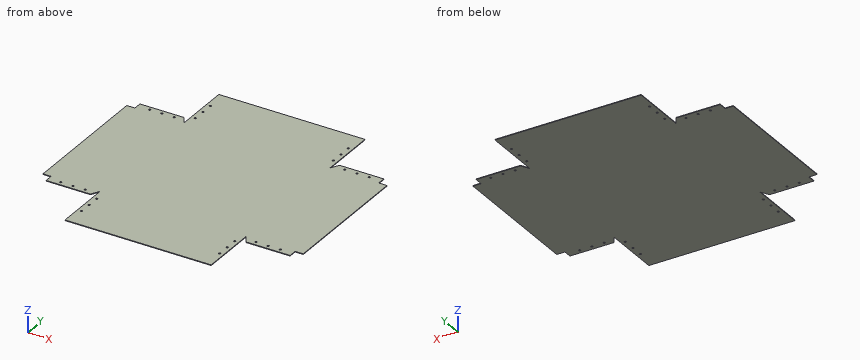
```python
from build123d import *

# Parameters (mm, degrees)
F0_W     = 227.80625
F0_H     = 12.7
F0_W_2   = 6.35
F0_H_2   = 212.725
F0_W_3   = 76.2
F0_R     = 1.5875
F1_DEPTH = 0.508


with BuildPart() as f1:
    # F0 (on Top) → F1 (new body, symmetric)
    with BuildSketch(Plane.XY):
        with Locations((0, -188.9125)):
            Rectangle(F0_W, F0_H)
        with Locations((-199.628125, 0)):
            Rectangle(F0_W_2, F0_H_2)
        with Locations((199.628125, 0)):
            Rectangle(F0_W_2, F0_H_2)
        Polygon((-107.553125, 182.5625), (113.903125, 182.5625), (113.903125, 195.2625), (-113.903125, 195.2625), (-113.903125, 182.5625), align=None)
        with Locations((-193.278125, 0)):
            Rectangle(F0_W_2, F0_H_2)
        with Locations((193.278125, 0)):
            Rectangle(F0_W_2, F0_H_2)
        with Locations((152.003125, 0)):
            Rectangle(F0_W_3, F0_H_2)
        with Locations((-152.003125, 0)):
            Rectangle(F0_W_3, F0_H_2)
        Polygon((-121.235473, -119.0625), (-113.903125, -106.3625), (-190.103125, -106.3625), (-190.103125, -119.0625), align=None)
        with Locations((-171.053125, -112.7125)):
            Circle(F0_R, mode=Mode.SUBTRACT)
        with Locations((-152.003125, -112.7125)):
            Circle(F0_R, mode=Mode.SUBTRACT)
        with Locations((-132.953125, -112.7125)):
            Circle(F0_R, mode=Mode.SUBTRACT)
        with BuildLine():
            Line((-131.365625, 112.7125), (-117.569299, 112.7125))
            Line((-117.569299, 112.7125), (-121.235473, 119.0625))
            Line((-121.235473, 119.0625), (-190.103125, 119.0625))
            Line((-190.103125, 119.0625), (-190.103125, 112.7125))
            Line((-190.103125, 112.7125), (-172.640625, 112.7125))
            ThreePointArc((-172.640625, 112.7125), (-171.053125, 114.3), (-169.465625, 112.7125))
            Line((-169.465625, 112.7125), (-153.590625, 112.7125))
            ThreePointArc((-153.590625, 112.7125), (-152.003125, 114.3), (-150.415625, 112.7125))
            Line((-150.415625, 112.7125), (-134.540625, 112.7125))
            ThreePointArc((-134.540625, 112.7125), (-132.953125, 114.3), (-131.365625, 112.7125))
        make_face()
        Polygon((190.103125, -106.3625), (113.903125, -106.3625), (121.235473, -119.0625), (190.103125, -119.0625), align=None)
        with Locations((132.953125, -112.7125)):
            Circle(F0_R, mode=Mode.SUBTRACT)
        with Locations((152.003125, -112.7125)):
            Circle(F0_R, mode=Mode.SUBTRACT)
        with Locations((171.053125, -112.7125)):
            Circle(F0_R, mode=Mode.SUBTRACT)
        Polygon((121.235473, 119.0625), (113.903125, 106.3625), (190.103125, 106.3625), (190.103125, 119.0625), align=None)
        with Locations((132.953125, 112.7125)):
            Circle(F0_R, mode=Mode.SUBTRACT)
        with Locations((152.003125, 112.7125)):
            Circle(F0_R, mode=Mode.SUBTRACT)
        with Locations((171.053125, 112.7125)):
            Circle(F0_R, mode=Mode.SUBTRACT)
        with BuildLine():
            Line((-190.103125, 106.3625), (-113.903125, 106.3625))
            Line((-113.903125, 106.3625), (-117.569299, 112.7125))
            Line((-117.569299, 112.7125), (-131.365625, 112.7125))
            ThreePointArc((-131.365625, 112.7125), (-132.953125, 111.125), (-134.540625, 112.7125))
            Line((-134.540625, 112.7125), (-150.415625, 112.7125))
            ThreePointArc((-150.415625, 112.7125), (-152.003125, 111.125), (-153.590625, 112.7125))
            Line((-153.590625, 112.7125), (-169.465625, 112.7125))
            ThreePointArc((-169.465625, 112.7125), (-171.053125, 111.125), (-172.640625, 112.7125))
            Line((-172.640625, 112.7125), (-190.103125, 112.7125))
            Line((-190.103125, 112.7125), (-190.103125, 106.3625))
        make_face()
        with BuildLine():
            Line((-113.903125, 106.3625), (-107.553125, 106.3625))
            Line((-107.553125, 106.3625), (-107.553125, 123.825))
            ThreePointArc((-107.553125, 123.825), (-109.140625, 125.4125), (-107.553125, 127))
            Line((-107.553125, 127), (-107.553125, 142.875))
            ThreePointArc((-107.553125, 142.875), (-109.140625, 144.4625), (-107.553125, 146.05))
            Line((-107.553125, 146.05), (-107.553125, 161.925))
            ThreePointArc((-107.553125, 161.925), (-109.140625, 163.5125), (-107.553125, 165.1))
            Line((-107.553125, 165.1), (-107.553125, 182.5625))
            Line((-107.553125, 182.5625), (-113.903125, 182.5625))
            Line((-113.903125, 182.5625), (-113.903125, 119.0625))
            Line((-113.903125, 119.0625), (-113.903125, 112.7125))
            Line((-113.903125, 112.7125), (-113.903125, 106.3625))
        make_face()
        Polygon((113.903125, -119.0625), (113.903125, -106.3625), (-113.903125, -106.3625), (-113.903125, -119.0625), (-113.903125, -182.5625), (113.903125, -182.5625), align=None)
        with Locations((-107.553125, -163.5125)):
            Circle(F0_R, mode=Mode.SUBTRACT)
        with Locations((-107.553125, -144.4625)):
            Circle(F0_R, mode=Mode.SUBTRACT)
        with Locations((-107.553125, -125.4125)):
            Circle(F0_R, mode=Mode.SUBTRACT)
        with Locations((107.553125, -163.5125)):
            Circle(F0_R, mode=Mode.SUBTRACT)
        with Locations((107.553125, -144.4625)):
            Circle(F0_R, mode=Mode.SUBTRACT)
        with Locations((107.553125, -125.4125)):
            Circle(F0_R, mode=Mode.SUBTRACT)
        with BuildLine():
            Line((-107.553125, 106.3625), (113.903125, 106.3625))
            Line((113.903125, 106.3625), (113.903125, 119.0625))
            Line((113.903125, 119.0625), (113.903125, 182.5625))
            Line((113.903125, 182.5625), (-107.553125, 182.5625))
            Line((-107.553125, 182.5625), (-107.553125, 165.1))
            ThreePointArc((-107.553125, 165.1), (-106.430593, 164.635032), (-105.965625, 163.5125))
            ThreePointArc((-105.965625, 163.5125), (-106.430593, 162.389968), (-107.553125, 161.925))
            Line((-107.553125, 161.925), (-107.553125, 146.05))
            ThreePointArc((-107.553125, 146.05), (-106.430593, 145.585032), (-105.965625, 144.4625))
            ThreePointArc((-105.965625, 144.4625), (-106.430593, 143.339968), (-107.553125, 142.875))
            Line((-107.553125, 142.875), (-107.553125, 127))
            ThreePointArc((-107.553125, 127), (-106.430593, 126.535032), (-105.965625, 125.4125))
            ThreePointArc((-105.965625, 125.4125), (-106.430593, 124.289968), (-107.553125, 123.825))
            Line((-107.553125, 123.825), (-107.553125, 106.3625))
        make_face()
        with Locations((107.553125, 125.4125)):
            Circle(F0_R, mode=Mode.SUBTRACT)
        with Locations((107.553125, 144.4625)):
            Circle(F0_R, mode=Mode.SUBTRACT)
        with Locations((107.553125, 163.5125)):
            Circle(F0_R, mode=Mode.SUBTRACT)
        Polygon((113.903125, -106.3625), (113.903125, 106.3625), (-107.553125, 106.3625), (-113.903125, 106.3625), (-113.903125, -106.3625), align=None)
    extrude(amount=F1_DEPTH, both=True)


solid = f1.part
```
Here's how the part is built. I have some questions about the finished solid (model axes, mm). Round coordinates to 2 decimals unless told otherwise and drop trailing zeros. Write each loop counter-clockwise with the first axis right and the second up, starting at its lowest first coordinate (ties: lowest second). Pieces come first, ordered by that corner, then holes.
Q1. If we section it at A-A on y = 172: Write out the boundary of the cut face in (x, z), plus the area to 3 significant figures.
Q2. If we section it at B-B on x = 164: Write out the boundary of the cut face in (y, z), plus the area to 3 significant figures.
Q3. If we section it at C-C on z = 0.35: Give the number of separate pieces and of enclosed holes in the cut face, plus the area to 3 significant figures.
Q4. Will these pins go through, and if not, where does the flat tip stop? P1, Ø5, axis at x = 107.55, y = -125.41, coming from the +Z side; P2, Ø0.5, axis at x = -154, z = 0, coming from the +Y side.
Q5. Please list where these lines run through material, in increasing order: probe 1 along Y at (x, z) = (-141, -0.35); probe 2 along X at (y, z) = (-130, -0.4).
Answer below:
1. outline: (-113.9, -0.51) - (113.9, -0.51) - (113.9, 0.51) - (-113.9, 0.51) - close
1. area: 231 mm2
2. outline: (-119.06, -0.51) - (119.06, -0.51) - (119.06, 0.51) - (-119.06, 0.51) - close
2. area: 242 mm2
3. separate pieces: 1
3. enclosed holes: 24
3. area: 130,000 mm2
4. P1: stops at z = 0.51
4. P2: stops at y = 119.06
5. probe 1: y = -119.06 to 119.06
5. probe 2: x = -113.9 to 113.9
